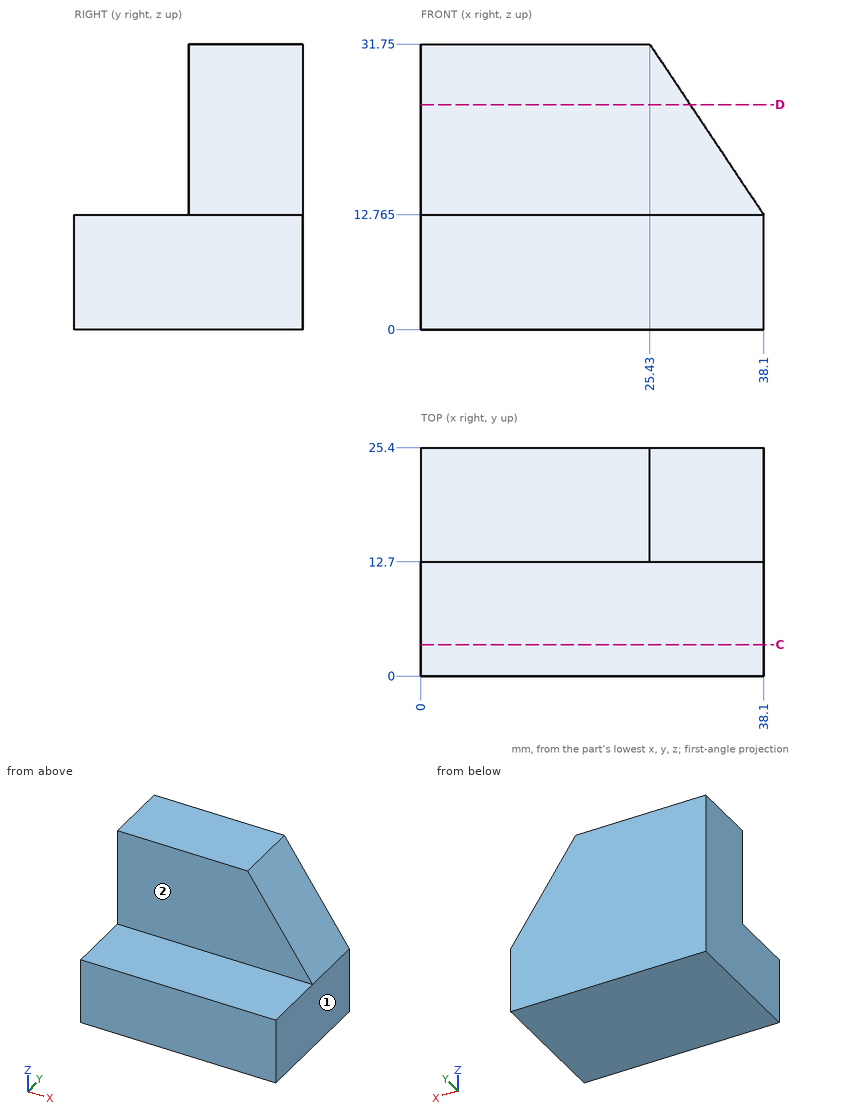
The drawing under review shows one solid part. Ordinate dimensions are in mm from its lowest x, y, z. A direction names the side the tool comes from. Give positions to 0.01 mm unless a question says otherwise; leave off trailing zeros. Write each loop counter-clockwise with the first axis right and the second up, starting at its lowest first coordinate (ties: lowest second). Pieces come first, ordered by that corner, then holes. Notation, with made-up numbers: (73.5, -7) - (99.5, -7) arc R24 cw to (99.5, 15) - close; hole circle Ø6 at (23, 1.25). An arc over 180 degrees is marked (long way). Answer in a Markdown table with one row per item. Add a question column.
1. Wall thickness on line 1 along Z through (x, y) = (36, 9.25) (1 decimal); line 2 along Y through (x, z) = (27, 14); line 3 along X through (y, z) = (14.5, 26.5) (1 decimal): over which ranges is each line inside the solid? List them lowest first. Write a range as [from, to].
2. Insertion check: P1, Ø15, axis at x = 23.5, z = 25.5, coming from the -Y side; P2, Ø6.5, axis at x = 12.5, y = 6.5, coming from the +Z side (1 decimal). Each pin has a flat end and moves straight along its axis. Give the tip position at first contact, or say it passes through.
3. We need section C-C on y = 3.5. Write out the cut boundary in (x, z) (1 decimal).
4. Tool access review of the marked faces 1 and 2: name each direction out of +Z, -Z, +X, -X, +Y, -Y from which nothing blocks a thin tool from reaching the whole face with its end or side.
5. We need section D-D on z = 25. Write out the cut boundary in (x, y) (1 decimal), then the cut area to 3 significant figures.
Ans:
| question | item | result |
|---|---|---|
| 1 | line 1 | z = [0, 12.8] |
| 1 | line 2 | y = [12.7, 25.4] |
| 1 | line 3 | x = [0, 28.9] |
| 2 | P1 | stops at y = 12.7 |
| 2 | P2 | stops at z = 12.8 |
| 3 | outline | (0, 0) - (38.1, 0) - (38.1, 12.8) - (0, 12.8) - close |
| 4 | face 1 | +Z, -Z, +X, +Y, -Y |
| 4 | face 2 | +Z, +X, -X, -Y |
| 5 | outline | (0, 12.7) - (29.9, 12.7) - (29.9, 25.4) - (0, 25.4) - close |
| 5 | area | 380 mm^2 |
